CAD build for the part. Positions are in the model's coordinates, mm. Face numbers are marked on the shaded views. A direction names the side the tool comes from. Coordinates: 2 decimals unless noted, no trailing zeros. Write each loop counter-clockwise with the first axis right and the second up, starting at its lowest first coordinate (ties: lowest second). Pieces come first, ordered by that corner, then holes. Notation, with made-up numbers: (-37.5, 47) -> (3.5, 47) arc R23 cw to (3.5, 66) -> close; hole circle Ø3 at (-14, 51.5). An arc over 180 degrees is marked (long way). Answer as CSV lines item,"result". Start each with the question number.
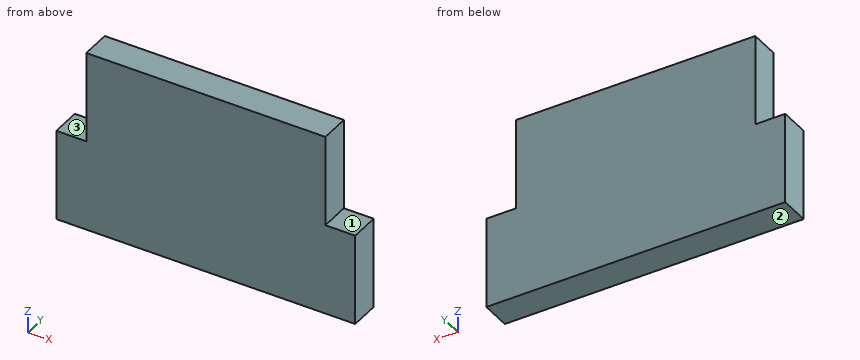
```python
from build123d import *

# Parameters (mm, degrees)
F0_W     = 20.32
F0_H     = 2.571502
F0_H_2   = 2.610788
F1_DEPTH = 2.54


with BuildPart() as f1:
    # F0 (on Front) → F1 (new body)
    with BuildSketch(Plane.XZ):
        Polygon((-74.706252, 3.87985), (-74.706252, 0), (-62.006252, 0), (-49.306252, 0), (-49.306252, 3.87985), align=None)
        Polygon((-74.706252, 7.7597), (-74.706252, 3.87985), (-49.306252, 3.87985), (-49.306252, 7.7597), (-51.841478, 7.7597), (-62.006252, 7.7597), (-72.161478, 7.7597), align=None)
        Polygon((-72.161478, 10.33711), (-72.161478, 7.7597), (-62.006252, 7.7597), (-51.841478, 7.7597), (-51.841478, 10.33711), align=None)
        with Locations((-62.001478, 11.622861)):
            Rectangle(F0_W, F0_H)
        with Locations((-62.001478, 14.214006)):
            Rectangle(F0_W, F0_H_2)
    extrude(amount=-F1_DEPTH)


solid = f1.part
```
1. Cut at B-B (x = -73). Give the cut face in (y, z).
2. Wall check: line 1 (X direction, y = 2.1, z = 9.25); line 2 (Z direction, x = -72.75, y = 1.9). Give the ranges that are in metal, low to high.
3. Cut at A-A (y = 2.3). Give the cut face in (x, z).
4. Tool access for the marked faces 1, 2 and 3: list every direction of +Z, -Z, +X, -X, +Y, -Y with a clear straight run to the whole face (end or side of a thin tool).
5. Cut at C-C (z = 9.75). Give the cut face in (x, y).
6. Flat gauge pins, fed straight in: P1, Ø6, axis at x = -63.5, z = 3.5, coming from the -Y side; P2, Ø1.3, axis at y = 1, z = 13.5, coming from the +X side; P3, Ø0.8, axis at x = -50.5, y = 1, coming from the +Z side. Where does each tip first touch, or does it go through?
Geometry check:
1,outline,"(0, 0) -> (2.54, 0) -> (2.54, 7.76) -> (0, 7.76) -> close"
2,line 1,"-72.16 to -51.84"
2,line 2,"0 to 7.76"
3,outline,"(-74.71, 0) -> (-49.31, 0) -> (-49.31, 7.76) -> (-51.84, 7.76) -> (-51.84, 15.52) -> (-72.16, 15.52) -> (-72.16, 7.76) -> (-74.71, 7.76) -> close"
4,face 1,"+Z, +X, +Y, -Y"
4,face 2,"-Z, +X, -X, +Y, -Y"
4,face 3,"+Z, -X, +Y, -Y"
5,outline,"(-72.16, 0) -> (-51.84, 0) -> (-51.84, 2.54) -> (-72.16, 2.54) -> close"
6,P1,"y = 0"
6,P2,"x = -51.84"
6,P3,"z = 7.76"
